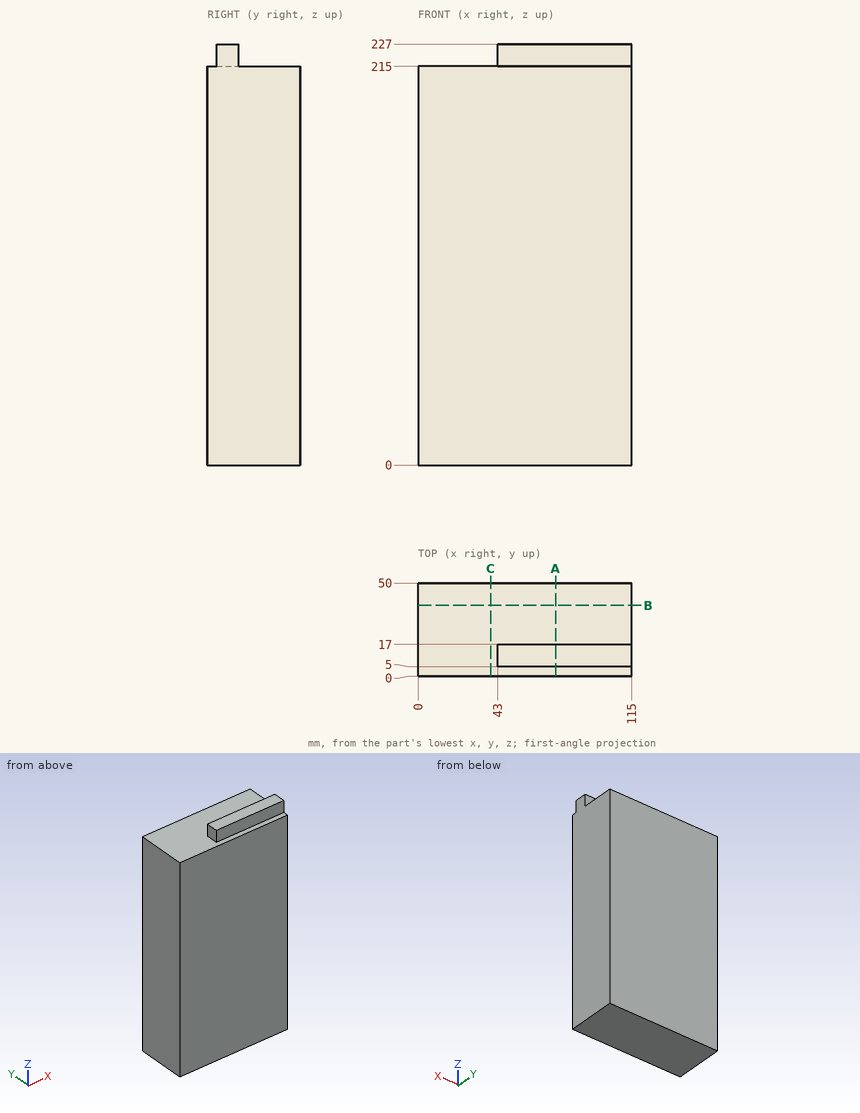
Answer from the drawing. Dimensions are ordinates in mm from the lowest x, y and z of the part. Round coordinates to 2 decimals unless told otherwise and drop trailing zeros. Order: outer loops, then holes, each group sorted by start corner. A loop starts at its lowest first (then second) coordinate and runs counter-clockwise, first axis right, second up. Notation, with made-up numbers: (-35.5, 19.5) - (-4.5, 19.5) arc R19 ccw to (-4.5, 55.5) - close; hole circle Ø8 at (60, -22). An arc over 180 degrees is marked (long way). Put each result on its own line as item: value. Start each with the question number.
(1) Find section C-C (x = 39). Give the vertices of the cut face in (y, z), plus the area to 4 significant figures.
(2) Find section B-B (y = 38). Give the vertices of the cut face in (x, z), plus the area to 3 significant figures.
(3) Find section A-A (x = 74). Give the vertices of the cut face in (y, z), plus the area to 3 significant figures.
(4) Given P1, Ø9.5, axis at x = 69, z = 221.5, coming from the +Y side; P2, Ø1.5, axis at x = 103, y = 33, coming from the +Z side, each flat-ended and moving along its own axis, determine where each tip first touches the part or whether it passes through.
(5) A straight line is drawn through the part: probe 1 along Z at (x, y) = (91, 24). Find the intervals that lie inside material, in ascending order. Write a range as from..to.
Reply:
1. outline: (0, 0) - (50, 0) - (50, 215) - (0, 215) - close
1. area: 10,750 mm^2
2. outline: (0, 0) - (115, 0) - (115, 215) - (0, 215) - close
2. area: 24,700 mm^2
3. outline: (0, 0) - (50, 0) - (50, 215) - (17, 215) - (17, 227) - (5, 227) - (5, 215) - (0, 215) - close
3. area: 10,900 mm^2
4. P1: y = 17
4. P2: z = 215
5. probe 1: 0..215
